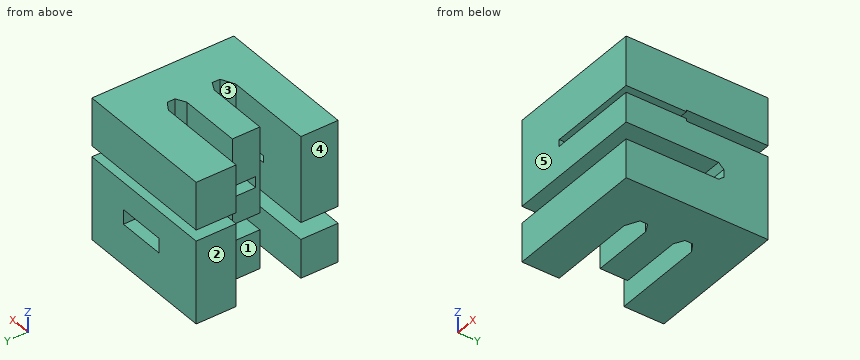
from build123d import *

# Parameters (mm, degrees)
F0_W     = 25
F0_H     = 25
F1_DEPTH = 25
F5_DEPTH = 32.1
F6_DEPTH = 40.6
F2_W     = 8.489821
F2_H     = 2.587373
F7_DEPTH = 45.1


with BuildPart() as f1:
    # F0 (on Top) → F1 (new body)
    with BuildSketch(Plane.XY):
        Rectangle(F0_W, F0_H)
    extrude(amount=F1_DEPTH)

    # F4 (on face) → F5 (intersect)
    with BuildSketch(Plane.XY.offset(25)):
        Polygon((12.5, 12.5), (-12.5, 12.5), (-12.5, 5.462941), (3.725921, 5.462941), (5.34303, 4.492676), (5.34303, 3.118134), (3.725921, 2.228724), (-7.189562, 2.228724), (-7.189562, -2.622602), (3.725921, -2.622602), (5.34303, -3.431156), (5.34303, -4.805698), (3.079078, -5.937674), (-12.5, -5.937674), (-12.5, -12.5), (12.5, -12.5), align=None)
    extrude(amount=-F5_DEPTH, mode=Mode.INTERSECT)

    # F3 (on face) → F6 (intersect)
    with BuildSketch(Plane.YZ.offset(12.5)):
        Polygon((12.5, 16.569659), (12.5, 25), (-12.5, 25), (-12.5, 9.823196), (3.778635, 9.823196), (4.693409, 8.965595), (4.693409, 7.593432), (3.778635, 6.850178), (-12.5, 6.850178), (-12.5, 0), (12.5, 0), (12.5, 14.625764), (-1.881534, 14.625764), (-1.881534, 16.569659), align=None)
    extrude(amount=-F6_DEPTH, mode=Mode.INTERSECT)

    # F2 (on face) → F7 (intersect)
    with BuildSketch(Plane.XZ.offset(12.5)):
        Polygon((12.5, 16.284853), (12.5, 25), (-12.5, 25), (-12.5, 0), (12.5, 0), (12.5, 15.072023), (-3.553276, 15.072023), (-3.553276, 16.284853), align=None)
        with Locations((0.691634, 8.522733)):
            Rectangle(F2_W, F2_H, mode=Mode.SUBTRACT)
    extrude(amount=-F7_DEPTH, mode=Mode.INTERSECT)


solid = f1.part
Could you check a few things on this model? Use its own coordinates, in mm. Face numbers are marked on the shaded views. A direction names the side the tool comes from. Coordinates: 2 decimals unless noted, no trailing zeros. Loops run counter-clockwise (first coordinate to the right, second up) from the corner with the lowest first, then second, coordinate; pieces in that order, holes last.
1. I need wall thicknesses on L1, parallel to Z at x = 2.5, y = 2; L2, parallel to Y at x = -0.5, z = 13; L3, parallel to Z at x = -2.25, y = 8.25. Which ranges of each line are inside material? Lowest first, please.
2. Imagine slicing it at A-A (y = 11.25). Please give me the cut outline in (x, z).
3. For the marked faces 1 and 2, which set-ups out of +Z, -Z, +X, -X, +Y, -Y let a thin tool reach every point of the face, with its end or its side?
4. Imagine slicing it at D-D (x = 9.5). Please give me the cut outline in (y, z), and give its area (3 significant figures).
5. Imagine slicing it at C-C (y = -1). Please give me the cut outline in (x, z), and give its area (3 significant figures).
6. Imagine slicing it at B-B (x = -9.5). Please give me the cut outline in (y, z), and give its area (3 significant figures).
7. We'd pull the mould along Y, two halves only. Please class the marked faces 3, 4 and 5: released by +Y, released by -Y, zero draft, split by the parting line, or undercut.
8. For P1, Ø1.5, axis at y = 4, z = 12, coming from the -X side; P2, Ø5.5, axis at y = 0, z = 4.5, coming from the -X side; P3, Ø0.7, axis at x = 8.5, z = 8.5, coming from the -Y side, each with a flat end and sliding along its axis, tell me the tip position at first contact or that it passes through.
Computed values:
1. L1: z = 0 to 6.85, 9.82 to 14.63, 16.57 to 25
1. L2: y = -12.5 to -5.94, -2.62 to 2.23, 5.46 to 12.5
1. L3: z = 0 to 7.23, 9.82 to 14.63, 16.57 to 25
2. outline: (-12.5, 0) - (12.5, 0) - (12.5, 14.63) - (-12.5, 14.63) - close; (-12.5, 16.57) - (12.5, 16.57) - (12.5, 25) - (-12.5, 25) - close; hole (-3.55, 7.23) - (4.94, 7.23) - (4.94, 9.82) - (-3.55, 9.82) - close
3. face 1: +Z, -Z, -X
3. face 2: +Z, -Z, -X, +Y, -Y
4. outline: (-12.5, 0) - (12.5, 0) - (12.5, 14.63) - (-1.88, 14.63) - (-1.88, 15.07) - (-12.5, 15.07) - (-12.5, 9.82) - (3.78, 9.82) - (4.69, 8.97) - (4.69, 7.59) - (3.78, 6.85) - (-12.5, 6.85) - close; (-12.5, 16.28) - (-1.88, 16.28) - (-1.88, 16.57) - (12.5, 16.57) - (12.5, 25) - (-12.5, 25) - close
4. area: 534 mm2
5. outline: (-7.19, 0) - (12.5, 0) - (12.5, 6.85) - (-7.19, 6.85) - close; (-7.19, 9.82) - (12.5, 9.82) - (12.5, 14.63) - (-7.19, 14.63) - close; (-7.19, 16.57) - (12.5, 16.57) - (12.5, 25) - (-7.19, 25) - close
5. area: 395 mm2
6. outline: (-12.5, 0) - (-5.94, 0) - (-5.94, 6.85) - (-12.5, 6.85) - close; (-12.5, 9.82) - (-5.94, 9.82) - (-5.94, 25) - (-12.5, 25) - close; (5.46, 0) - (12.5, 0) - (12.5, 14.63) - (5.46, 14.63) - close; (5.46, 16.57) - (12.5, 16.57) - (12.5, 25) - (5.46, 25) - close
6. area: 307 mm2
7. face 3: undercut
7. face 4: zero draft
7. face 5: released by -Y
8. P1: stops at x = 4.91
8. P2: stops at x = -7.19
8. P3: stops at y = 4.69
